Autodesk Inventor part; units mm, degrees
ref_plane "YZ Plane" through (0, 0, 0) normal (1, 0, 0) x (0, 1, 0)
ref_plane "XZ Plane" through (0, 0, 0) normal (0, 1, 0) x (-1, 0, 0)
ref_plane "XY Plane" through (0, 0, 0) normal (0, 0, 1) x (1, 0, 0)
ref_plane "Work Plane2" through (-37.9568, -6.3739, 16.6205) normal (0.2239, -0.0206, 0.9744) x (0.9746, 0.0023, -0.2239)
sketch "Sketch1" plane through (-37.9568, -6.3739, 16.6205) normal (0.2239, -0.0206, 0.9744) x (0.9746, 0.0023, -0.2239)
  circle A0 centre (40.7292, 6.1193) radius 2.5
  line L0 (45.348, 6.1193) -> (43.0386, 2.1193)
  line L1 (43.0386, 2.1193) -> (38.4198, 2.1193)
  line L2 (38.4198, 2.1193) -> (36.1104, 6.1193)
  line L3 (36.1104, 6.1193) -> (38.4198, 10.1193)
  line L4 (38.4198, 10.1193) -> (43.0386, 10.1193)
  line L5 (43.0386, 10.1193) -> (45.348, 6.1193)
  point P0 (40.7292, 6.1193)
  dimension "d0" = 5
  dimension "d1" = 8
extrude "Extrusion1" add sketch "Sketch1" along normal blind 4
properties part number "m5_nut"
The model under review builds one solid part; all positions refer to its coordinate system, in mm. Round coordinates to 2 decimals unless told otherwise and drop trailing zeros. Loops run counter-clockwise (first coordinate to the right, second up) from the corner with the lowest first, then second, coordinate; pieces in that order, holes last. Notation, with made-up numbers: M 85,31.5 L 111,31.5 A29 ccw 111,60.5 Z; hole C 63.25,46 d6. An arc over 180 degrees is marked long. Write item = value, one per line.
Item 1: Take a section at B-B on x = 6.75. Write out the cut boundary in (y, z), then the cut area to 3 significant figures.
Return value:
outline = M -0.94,10.57 L -0.2,8.75 L 0.48,10.6 Z
area = 1.30 mm2
Item 2: For line 1 (X direction, y = -1.75, z = 9.8); line 2 (Y direction, x = 3.75, z = 9.2); line 3 (Y direction, x = 0.75, z = 8.65), list the stretches that pass through material, from the lowest coordinate up. Write a range as [from, to].
Return value:
line_1 = [-1.56, 0.24], [4.28, 6.09]
line_2 = [-4.2, -2.13], [1.72, 3.8]
line_3 = [-4.18, -2.37], [2.01, 3.82]
Item 3: The part is to be moulded in two halves that separate along Y. For faces 1 (the flat face through (-1.193, 1.761, 10.369)), 2 (the cylindrical face through (4.517, -0.948, 8.999)), 3 (the flat face through (5.58, -2.17, 8.73)), say which applies: released by +Y, released by -Y, zero draft, split by the parting line, or undercut.
Return value:
face_1 = released by +Y
face_2 = undercut
face_3 = released by -Y
Item 4: Insertion check: P1, Ø1.5, axis at x = -1.5, z = 10.5, coming from the +Y side; P2, Ø1.5, axis at x = 5.5, z = 11, coming from the -Y side. Each pin has a flat end and moves straight along its axis. Give the tip position at first contact, or say it passes through.
Return value:
P1 = 2.49
P2 = -4.24
Item 5: Take a section at C-C on y = 2.75. Write out the cut boundary in (x, z), then the cut area to 3 significant figures.
Return value:
outline = M -1.1,8.34 L 4.63,7.03 L 5.48,10.94 L -0.16,12.23 Z
area = 23.3 mm2
Item 6: Take a section at A-A on y = -3. Write out the cut boundary in (x, z).
Return value:
outline = M -1.16,8.24 L 4.65,6.9 L 5.59,10.79 L -0.31,12.15 Z
